```python
from build123d import *

# Parameters (mm, degrees)
SKETCH1_W               = 81
SKETCH1_H               = 57
BOSS_EXTRUDE1_DEPTH     = 43
CUT_EXTRUDE1_DEPTH      = 87.180044094
CUT_EXTRUDE1_DEPTH_BACK = 87.180044094
CUT_EXTRUDE2_DEPTH      = 87.180044094
CUT_EXTRUDE2_DEPTH_BACK = 87.180044094
SKETCH3_W               = 56.062487614
SKETCH3_H               = 49.157310494
CUT_EXTRUDE4_DEPTH      = 87.180044094
CUT_EXTRUDE4_DEPTH_BACK = 87.180044094
SKETCH4_R               = 7
FILLET1_R               = 5
CUT_EXTRUDE5_DEPTH      = 87.180044094
CUT_EXTRUDE5_DEPTH_BACK = 87.180044094
CUT_EXTRUDE7_DEPTH      = 87.180044094
CUT_EXTRUDE7_DEPTH_BACK = 87.180044094
SKETCH6_R               = 19
CUT_EXTRUDE8_DEPTH      = 87.180044094
CUT_EXTRUDE8_DEPTH_BACK = 87.180044094


with BuildPart() as part:
    # Sketch1 → Boss-Extrude1 (new body)
    with BuildSketch(Plane.XY):
        with Locations((26.5, -4.5)):
            Rectangle(SKETCH1_W, SKETCH1_H)
    extrude(amount=BOSS_EXTRUDE1_DEPTH)

    # Sketch2 → Cut-Extrude1 (cut, two sides: drawn at the far end of the back side and taken through both)
    with BuildSketch(Plane.XY.offset(-CUT_EXTRUDE1_DEPTH_BACK)):
        Polygon((38, -33), (67, 0), (92.563073461, 0), (92.563073461, -46.247191662), (38, -46.247191662), align=None)
    extrude(amount=CUT_EXTRUDE1_DEPTH + CUT_EXTRUDE1_DEPTH_BACK, mode=Mode.SUBTRACT)

    # Sketch3 → Cut-Extrude2 (cut, two sides: drawn at the far end of the back side and taken through both)
    with BuildSketch(Plane.XY.offset(-CUT_EXTRUDE2_DEPTH_BACK)):
        Polygon((67, 19), (62, 24), (62, 35.07400688), (76.394076925, 35.07400688), (76.394076925, 19), align=None)
        with Locations((-2.33427411, -38.578655247)):
            Rectangle(SKETCH3_W, SKETCH3_H)
    extrude(amount=CUT_EXTRUDE2_DEPTH + CUT_EXTRUDE2_DEPTH_BACK, mode=Mode.SUBTRACT)

    # Sketch4 → Cut-Extrude4 (cut, two sides: drawn at the far end of the back side and taken through both)
    with BuildSketch(Plane.XY.offset(-CUT_EXTRUDE4_DEPTH_BACK)):
        Circle(SKETCH4_R)
        Polygon((-14, -7), (-7, -14), (-7, -25.581490966), (-25.698807285, -25.581490966), (-25.698807285, 4.698807285), align=None)
        with BuildLine():
            Line((25.696969697, -14), (1.830031376, -60.145765031))
            Line((1.830031376, -60.145765031), (54.696969697, -43))
            ThreePointArc((54.696969697, -43), (34.190873043, -34.506096654), (25.696969697, -14))
        make_face()
    extrude(amount=CUT_EXTRUDE4_DEPTH + CUT_EXTRUDE4_DEPTH_BACK, mode=Mode.SUBTRACT)

    # Fillet1
    fillet1_edges = [part.edges().sort_by_distance(p)[0] for p in [
        (25.696969697, -14, 21.5),
    ]]
    fillet(fillet1_edges, radius=FILLET1_R)

    # Sketch5 → Cut-Extrude5 (cut, two sides: drawn at the far end of the back side and taken through both)
    with BuildSketch(Plane.XY.offset(-CUT_EXTRUDE5_DEPTH_BACK)):
        Polygon((-14, 17), (-7, 24), (-7, 33.910955106), (-24.773301804, 33.910955106), (-24.773301804, 17), align=None)
    extrude(amount=CUT_EXTRUDE5_DEPTH + CUT_EXTRUDE5_DEPTH_BACK, mode=Mode.SUBTRACT)

    # Sketch6 → Cut-Extrude7 (cut, two sides: drawn at the far end of the back side and taken through both)
    with BuildSketch(Plane.XY.offset(-CUT_EXTRUDE7_DEPTH_BACK)):
        with Locations((25.977509097, 38.71256988)):
            Circle(SKETCH6_R)
    extrude(amount=CUT_EXTRUDE7_DEPTH + CUT_EXTRUDE7_DEPTH_BACK, mode=Mode.SUBTRACT)

    # Sketch7 → Cut-Extrude8 (cut, two sides: drawn at the far end of the back side and taken through both)
    with BuildSketch(Plane.XY.offset(-CUT_EXTRUDE8_DEPTH_BACK)):
        with BuildLine():
            Line((13.955018194, 24), (0, 24))
            Line((0, 24), (22.678193721, 20.001222573))
            ThreePointArc((22.678193721, 20.001222573), (18.059997358, 21.440829729), (13.955018194, 24))
        make_face()
    extrude(amount=CUT_EXTRUDE8_DEPTH + CUT_EXTRUDE8_DEPTH_BACK, mode=Mode.SUBTRACT)


solid = part.part
```
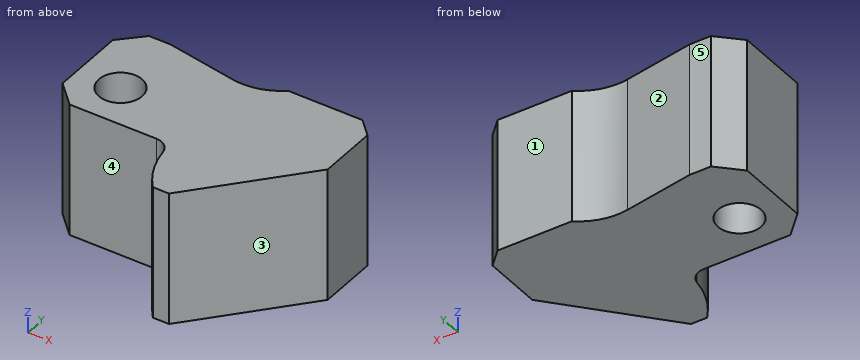
Can you work these out from the model? Positions are in its coordinate system, mm. Face numbers are marked on the shaded views. A direction names the side the tool comes from. Coordinates: 2 decimals unless noted, no trailing zeros. Loops run counter-clockwise (first coordinate to the right, second up) from the corner with the lowest first, then second, coordinate; pieces in that order, holes last. Notation, with made-up numbers: (32.5, 44) -> (73.5, 44) arc R18 ccw to (73.5, 68) -> close; hole circle Ø1 at (30, 59.5). An arc over 180 degrees is marked (long way). Answer as a JSON object with one key per item and string values.
1) Imagine slicing it at A-A (z = 31.5). Please give me the cut outline in (x, y), then the cut area to 3 significant figures.
Results:
{"outline": "(-14, -7) -> (-7, -14) -> (21.07, -14) arc R5 cw to (26.01, -18.26) arc R29 ccw to (32.79, -33) -> (38, -33) -> (67, 0) -> (67, 19) -> (62, 24) -> (38, 24) arc R19 cw to (22.68, 20) -> (0, 24) -> (-7, 24) -> (-14, 17) -> close; hole circle Ø14 at (0, 0)", "area": "3,040 mm^2"}
2) Imagine slicing it at C-C (y = -26.5). Please give me the cut outline in (x, z), then the cut area to 3 significant figures.
Results:
{"outline": "(28.53, 0) -> (43.71, 0) -> (43.71, 43) -> (28.53, 43) -> close", "area": "653 mm^2"}
3) For the marked faces 4 and 5, which set-ups out of +Z, -Z, +X, -X, +Y, -Y let a thin tool reach every point of the face, with its end or its side?
Results:
{"face 4": "+Z, -Z, -X, -Y", "face 5": "+Z, -Z, +X, -X, +Y"}
4) Thinking about a two-plate mould opening in X: for the marked faces 1, 2 and 3, which applies, pulls with the +X half, pulls with the -X half, needs draft (parallel to the pull), parting line crosses it, or undercut?
Results:
{"face 1": "needs draft", "face 2": "undercut", "face 3": "pulls with the +X half"}
5) For P1, Ø3, axis at x = 16.5, z = 33.5, coming from the +Y side; P2, Ø11, axis at x = 0, y = 0, coming from the -Z side; P3, Ø22.5, axis at x = 14, z = 26, coming from the -Y side; P4, Ø2, axis at x = 48.5, z = 20, coming from the -Y side, each with a flat end and sliding along its axis, tell me the tip position at first contact or that it passes through.
Results:
{"P1": "stops at y = 21.36", "P2": "passes through", "P3": "stops at y = -16.26", "P4": "stops at y = -22.19"}
6) If I drill on line 1 (X direction, y = 0, z = 32.5); line 2 (Y direction, x = 0, z = 14); line 3 (X direction, y = 2, z = 33), over which ranges is the centre line in solid material (lowest first)?
Results:
{"line 1": "x = -14 to -7, 7 to 67", "line 2": "y = -14 to -7, 7 to 24", "line 3": "x = -14 to -6.71, 6.71 to 67"}
7) Imagine slicing it at B-B (x = 54). Please give me the cut outline in (y, z).
Results:
{"outline": "(-14.79, 0) -> (24, 0) -> (24, 43) -> (-14.79, 43) -> close"}
